Design review of the part built by this model. Coordinates are the model's own, in mm. A direction names the side the tool comes from. Give positions to 0.01 mm unless a question says otherwise; leave off trailing zeros. Write each loop counter-clockwise with the first axis right and the second up, starting at its lowest first coordinate (ties: lowest second). Pieces come first, ordered by that corner, then holes. Notation, with made-up numbers: M -5.5,-15.75 L 9.5,-15.75 A32 cw 9.5,21.25 Z; hole C 0.25,43.5 d10. An arc over 180 degrees is marked long. Answer in a Markdown table with one row per item.
```python
from build123d import *

# Parameters (mm, degrees)
F0_W     = 52
F0_H     = 42
F0_W_2   = 42
F0_H_2   = 32
F1_DEPTH = 3
F2_R     = 5
F3_SIZE2 = 1
F3_SIZE  = 1
F4_SIZE  = 1
F5_SIZE  = 0.1


with BuildPart() as f1:
    # F0 (on Top) → F1 (new body)
    with BuildSketch(Plane.XY):
        Rectangle(F0_W, F0_H)
        Rectangle(F0_W_2, F0_H_2, mode=Mode.SUBTRACT)
    extrude(amount=F1_DEPTH)

    # F2
    f2_edges = [f1.edges().sort_by_distance(p)[0] for p in [
        (-26, 21, 1.5),
        (-26, -21, 1.5),
        (26, -21, 1.5),
        (26, 21, 1.5),
    ]]
    fillet(f2_edges, radius=F2_R)

    # F3
    f3_edges = [f1.edges().sort_by_distance(p)[0] for p in [
        (-21, 16, 1.5),
    ]]
    chamfer(f3_edges, length=F3_SIZE, length2=F3_SIZE2)

    # F4
    f4_edges = [f1.edges().sort_by_distance(p)[0] for p in [
        (21, 16, 1.5),
        (21, -16, 1.5),
        (-21, -16, 1.5),
    ]]
    chamfer(f4_edges, length=F4_SIZE)

    # F5
    f5_edges = [f1.edges().sort_by_distance(p)[0] for p in [
        (-21, 0, 3),
        (-20.5, -15.5, 3),
        (-20.5, 15.5, 3),
        (0, -16, 3),
        (0, 16, 3),
        (20.5, -15.5, 3),
        (20.5, 15.5, 3),
        (21, 0, 3),
        (0, 21, 3),
        (24.535534, 19.535534, 3),
        (-24.535534, 19.535534, 3),
        (26, 0, 3),
        (-26, 0, 3),
        (24.535534, -19.535534, 3),
        (-24.535534, -19.535534, 3),
        (0, -21, 3),
        (-21, 0, 0),
        (-20.5, -15.5, 0),
        (-20.5, 15.5, 0),
        (0, -16, 0),
        (0, 16, 0),
        (20.5, -15.5, 0),
        (20.5, 15.5, 0),
        (21, 0, 0),
        (0, 21, 0),
        (24.535534, 19.535534, 0),
        (-24.535534, 19.535534, 0),
        (26, 0, 0),
        (-26, 0, 0),
        (24.535534, -19.535534, 0),
        (-24.535534, -19.535534, 0),
        (0, -21, 0),
    ]]
    chamfer(f5_edges, length=F5_SIZE)


solid = f1.part
```
1) For faces 4 (the face through (24, -20, 2)), 5 (the face through (0, -16, 1)), list the 3-axis set-ups (+Z, -Z, +X, -X, +Y, -Y) from which the entire face can be reached by the end or side of a thin tool; tool diameter is ignored.
Geometry says:
| item | result |
|---|---|
| face 4 | +Z, -Z, +X, -Y |
| face 5 | +Z, -Z |
2) To check wall thickness, follow probe 1 along Y at (x, z) = (2, 1.6); probe 2 along X at (y, z) = (-6.5, 0.4); probe 3 along Y at (x, z) = (22, 1.8). State the ranges of each line that lie inside material, in increasing order. Write a range as [from, to].
Geometry says:
| item | result |
|---|---|
| probe 1 | [-21, -16], [16, 21] |
| probe 2 | [-26, -21], [21, 26] |
| probe 3 | [-20.9, 20.9] |
3) Add section C-C (z = 1.6). Write out the cut boundary in (x, y), and give its area (3 significant figures).
Geometry says:
| item | result |
|---|---|
| outline | M -26,-16 A5 ccw -21,-21 L 21,-21 A5 ccw 26,-16 L 26,16 A5 ccw 21,21 L -21,21 A5 ccw -26,16 Z; hole M -21,-15 L -20,-16 L 20,-16 L 21,-15 L 21,15 L 20,16 L -20,16 L -21,15 Z |
| area | 821 mm^2 |
4) Add section B-B (x = 13). Write out the cut boundary in (y, z), and give its area (3 significant figures).
Geometry says:
| item | result |
|---|---|
| outline | M -21,0.1 L -20.9,0 L -16.1,0 L -16,0.1 L -16,2.9 L -16.1,3 L -20.9,3 L -21,2.9 Z; M 16,0.1 L 16.1,0 L 20.9,0 L 21,0.1 L 21,2.9 L 20.9,3 L 16.1,3 L 16,2.9 Z |
| area | 30.0 mm^2 |
5) Add section A-A (y = -10). Write out the cut boundary in (x, z), and give its area (3 significant figures).
Geometry says:
| item | result |
|---|---|
| outline | M -26,0.1 L -25.9,0 L -21.1,0 L -21,0.1 L -21,2.9 L -21.1,3 L -25.9,3 L -26,2.9 Z; M 21,0.1 L 21.1,0 L 25.9,0 L 26,0.1 L 26,2.9 L 25.9,3 L 21.1,3 L 21,2.9 Z |
| area | 30.0 mm^2 |
6) The part is to be moulded in two halves that separate along Y. For faces 1 (the face through (-26, 0, 1)), 2 (the face through (-25, -19, 2)), 3 (the face through (0, 16, 1)), say which applies: released by +Y, released by -Y, zero draft, split by the parting line, or undercut.
Geometry says:
| item | result |
|---|---|
| face 1 | zero draft |
| face 2 | released by -Y |
| face 3 | undercut |
